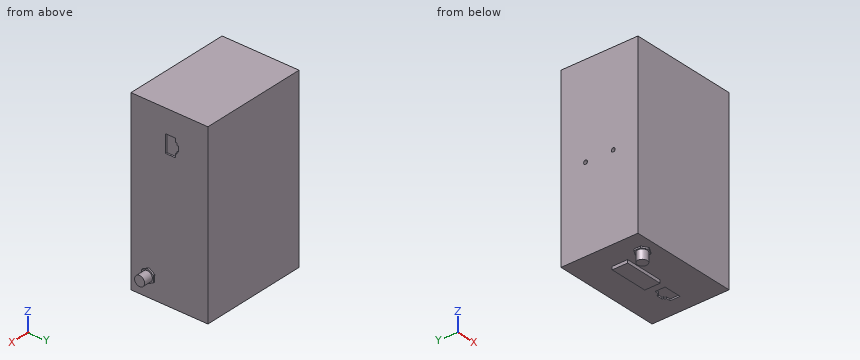
from build123d import *

# Parameters (mm, degrees)
SKETCH_1_W             = 70
SKETCH_1_H             = 50
EXTRUDE_1_DEPTH        = 115
CUT_EXTRUDE_1_DEPTH    = 1
EXTRUDE_2_DEPTH        = 1
SKETCH_4_R             = 3.25
EXTRUDE_3_DEPTH        = 6
EXTRUDE_4_DEPTH        = 1
SKETCH_6_R             = 3.25
EXTRUDE_5_DEPTH        = 6
CUT_EXTRUDE_2_DEPTH    = 1
HOLE_WIZARD_M3_1_D     = 2.5
HOLE_WIZARD_M3_1_DEPTH = 2
HOLE_WIZARD_M3_1_TIP   = 0.751075774
SKETCH_10_W            = 25
SKETCH_10_H            = 10
EXTRUDE_6_DEPTH        = 2


with BuildPart() as part:
    # 草图1 → 凸台-拉伸1 (new body)
    with BuildSketch(Plane.XY):
        Rectangle(SKETCH_1_W, SKETCH_1_H)
    extrude(amount=EXTRUDE_1_DEPTH)

    # 草图2 → 切除-拉伸1 (cut)
    with BuildSketch(Plane(origin=(35, 0, 0), x_dir=(0, 0, -1), z_dir=(1, 0, 0))):
        Polygon((-100, -2.5), (-88.5, -2.5), (-88.5, 4), (-91, 4), (-91, 5), (-92.5, 5), (-92.5, 6), (-96, 6), (-96, 5), (-97.5, 5), (-97.5, 4), (-100, 4), align=None)
    extrude(amount=-CUT_EXTRUDE_1_DEPTH, mode=Mode.SUBTRACT)

    # 草图3 → 凸台-拉伸2 (add)
    with BuildSketch(Plane(origin=(35, 0, 0), x_dir=(0, 0, -1), z_dir=(1, 0, 0))):
        Polygon((-15.124996356, -9.533340135), (-17.49772639, -13.356970895), (-15.372730033, -17.32363076), (-10.875003644, -17.466659865), (-8.50227361, -13.643029105), (-10.627269967, -9.67636924), align=None)
    extrude(amount=EXTRUDE_2_DEPTH)

    # 草图4 → 凸台-拉伸3 (add)
    with BuildSketch(Plane(origin=(36, 0, 0), x_dir=(0, 0, -1), z_dir=(1, 0, 0))):
        with Locations((-13, -13.5)):
            Circle(SKETCH_4_R)
    extrude(amount=EXTRUDE_3_DEPTH)

    # 草图5 → 凸台-拉伸4 (add)
    with BuildSketch(Plane(origin=(0, 0, 0), x_dir=(-1, 0, 0), z_dir=(0, 0, -1))):
        Polygon((24.897114317, -18.25), (24.897114317, -13.75), (21, -11.5), (17.102885683, -13.75), (17.102885683, -18.25), (21, -20.5), align=None)
    extrude(amount=EXTRUDE_4_DEPTH)

    # 草图6 → 凸台-拉伸5 (add)
    with BuildSketch(Plane(origin=(0, 0, -1), x_dir=(-1, 0, 0), z_dir=(0, 0, -1))):
        with Locations((21, -16)):
            Circle(SKETCH_6_R)
    extrude(amount=EXTRUDE_5_DEPTH)

    # 草图7 → 切除-拉伸2 (cut)
    with BuildSketch(Plane(origin=(0, 0, 0), x_dir=(-1, 0, 0), z_dir=(0, 0, -1))):
        Polygon((-24, 4), (-21.25, 4), (-21.25, 5), (-20.25, 5), (-20.25, 6), (-16.25, 6), (-16.25, 5), (-15.25, 5), (-15.25, 4), (-12.5, 4), (-12.5, -2.5), (-24, -2.5), align=None)
    extrude(amount=-CUT_EXTRUDE_2_DEPTH, mode=Mode.SUBTRACT)

    # M3 螺纹孔的螺纹孔钻头1
    with Locations(Plane.ZY.offset(35)):
        with Locations((55, -9), (55, 9)):
            Hole(HOLE_WIZARD_M3_1_D / 2, depth=HOLE_WIZARD_M3_1_DEPTH)
            with Locations((0, 0, -(HOLE_WIZARD_M3_1_DEPTH + HOLE_WIZARD_M3_1_TIP / 2))):  # 118° drill point
                Cone(0, HOLE_WIZARD_M3_1_D / 2, HOLE_WIZARD_M3_1_TIP, mode=Mode.SUBTRACT)

    # 草图10 → 凸台-拉伸6 (add)
    with BuildSketch(Plane(origin=(0, 0, 0), x_dir=(-1, 0, 0), z_dir=(0, 0, -1))):
        with Locations((6.785143616, 0)):
            Rectangle(SKETCH_10_W, SKETCH_10_H)
    extrude(amount=EXTRUDE_6_DEPTH)


solid = part.part
Read the model definition and answer for the solid it produces. Units are mm, in the model's axes. Give positions to 0.01 mm unless a question says otherwise; leave off trailing zeros. Write each loop counter-clockwise with the first axis right and the second up, starting at its lowest first coordinate (ties: lowest second). Pieces come first, ordered by that corner, then holes. Notation, with made-up numbers: (75, 74) - (119, 74) arc R13 ccw to (119, 91) - close; hole circle Ø5 at (16.25, 36). An arc over 180 degrees is marked (long way). Answer in a Markdown table with one row per item. Add a question column.
Item 1: Section A-A, the plane z = 94.5 is taken. Write down the section's boundary in (x, y), and give its area (3 significant figures).
Item 2: Flat-ended cylindrical pins translate along their axes: P1, Ø2.5, axis at y = 0, z = 95, coming from the +X side; P2, Ø0.8, axis at y = 5.5, z = 0.5, coming from the +X side; P3, Ø10, axis at x = -3.5, y = 4, coming from the -Z side. Find the tip coordinate at first contact, or state that the pin passes through.
Item 3: Section C-C, the plane y = 16.5 is taken. Write down the section's boundary in (x, z), and give its area (3 significant figures).
Item 4: Find the intervals of material crossed by L1, parallel to Y at x = -34.4, z = 55; L2, parallel to Z at x = -34.1, y = 9; L3, parallel to X at y = 3, z = 69.5, in increasing order.
Item 5: Section D-D, the plane z = 79 is taken. Write down the section's boundary in (x, y).
Item 6: Section B-B, the plane x = -5.5 is taken. Write down the section's boundary in (y, z), and give its area (3 significant figures).
Recorded:
| question | item | result |
|---|---|---|
| 1 | outline | (-35, -25) - (35, -25) - (35, -2.5) - (34, -2.5) - (34, 6) - (35, 6) - (35, 25) - (-35, 25) - close |
| 1 | area | 3,490 mm2 |
| 2 | P1 | stops at x = 34 |
| 2 | P2 | stops at x = 35 |
| 2 | P3 | stops at z = -2 |
| 3 | outline | (-35, 0) - (35, 0) - (35, 115) - (-35, 115) - close |
| 3 | area | 8,050 mm2 |
| 4 | L1 | y = -25 to -10.25, -7.75 to 7.75, 10.25 to 25 |
| 4 | L2 | z = 0 to 53.75, 56.25 to 115 |
| 4 | L3 | x = -35 to 35 |
| 5 | outline | (-35, -25) - (35, -25) - (35, 25) - (-35, 25) - close |
| 6 | outline | (-25, 0) - (-5, 0) - (-5, -2) - (5, -2) - (5, 0) - (25, 0) - (25, 115) - (-25, 115) - close |
| 6 | area | 5,770 mm2 |
